Work out the finished part from the listing and answer in its coordinate system (mm). Give positions to 0.01 mm unless a question says otherwise; leave off trailing zeros. Loops run counter-clockwise (first coordinate to the right, second up) from the corner with the lowest first, then second, coordinate; pieces in that order, holes last. Notation, with made-up numbers: (28.5, 62.5) - (82.5, 62.5) arc R8 ccw to (82.5, 71.5) - close; hole circle Ø8 at (54.25, -30). An arc over 180 degrees is marked (long way). One line per question, with ' | ' between items.
Autodesk Inventor part; units mm, degrees
ref_plane "Work Plane1" through (9.2075, 0, 0) normal (1, 0, 0) x (0, 0, -1)
ref_plane "YZ Plane" through (0, 0, 0) normal (1, 0, 0) x (0, 1, 0)
ref_plane "XZ Plane" through (0, 0, 0) normal (0, 1, 0) x (-1, 0, 0)
sketch "Sketch1" plane through (0, 0, 0) normal (1, 0, 0) x (0, 1, 0)
  line L0 (147.32, 113.03) -> (-147.32, 113.03)
  line L1 (-147.32, 113.03) -> (-147.32, -113.03)
  line L2 (-147.32, -113.03) -> (147.32, -113.03)
  line L3 (147.32, -113.03) -> (147.32, 113.03)
  line L4 (147.32, 113.03) -> (-147.32, -113.03) construction
  line L5 (-147.32, 113.03) -> (147.32, -113.03) construction
  point P0 (0, 0)
  dimension "d0" = 294.64
  dimension "d1" = 226.06
extrude "Extrusion1" add sketch "Sketch1" along normal blind 2.8575
sketch "Sketch2" plane through (2.8575, 0, 0) normal (1, 0, 0) x (0, 0, -1)
  line L0 (113.03, 60.96) -> (100.33, 60.96)
  line L1 (100.33, 60.96) -> (100.33, -46.99)
  line L2 (100.33, -46.99) -> (113.03, -46.99)
  line L3 (113.03, -147.32) -> (113.03, 147.32)
  line L4 (113.03, 147.32) -> (-113.03, 147.32)
  line L5 (113.03, 60.96) -> (113.03, -46.99)
  point P0 (0, 0)
  dimension "d4" = 107.95
  dimension "d5" = 0
  dimension "d6" = 0
  dimension "d7" = 12.7
  dimension "d8" = 86.36
extrude "Extrusion2" cut sketch "Sketch2" against normal blind 2.8575
mirror "Mirror1" about plane through (0, 0, 0) normal (0, 0, 1) of "Extrusion2"
ref_plane "Work Plane1" through (9.2075, 0, 0) normal (1, 0, 0) x (0, 0, -1)
fillet "Fillet2" radius 0.762 12 edges at (0, 104.14, -113.03) (0, 6.985, -100.33) (0, 60.96, -106.68) (0, -97.155, -113.03) (0, -46.99, -106.68) (0, -147.32, 0) (0, -97.155, 113.03) (0, -46.99, 106.68) (0, 6.985, 100.33) (0, 60.96, 106.68) (0, 104.14, 113.03) (2.8575, 147.32, 0)
fillet "Fillet4" radius 0.254 18 edges at (2.8575, -147.32, 0) (2.8575, -97.155, -113.03) (2.8575, 6.985, -100.33) (2.8575, -46.99, -106.68) (2.6343, 147.0968, -113.03) (1.4287, 147.32, -113.03) (0.2232, 147.32, -112.8068) (0, 147.32, 0) (0.2232, 147.32, 112.8068) (1.4287, 147.32, 113.03) (2.6343, 147.0968, 113.03) (2.8575, 103.759, 113.03) (2.8575, 103.759, -113.03) (2.8575, 60.96, -106.68) (2.8575, 60.96, 106.68) (2.8575, 6.985, 100.33) (2.8575, -97.155, 113.03) (2.8575, -46.99, 106.68)
sketch "Sketch7" plane through (0, 0, 0) normal (-1, 0, 0) x (0, 0, 1)
  circle A0 centre (-13.97, -138.938) radius 2.54
  line L0 (0, 0) -> (0, -146.558) construction
  line L1 (112.268, -146.558) -> (-112.268, -146.558)
  circle A1 centre (13.97, -138.938) radius 2.54
  dimension "d22" = 5.08
  dimension "d23" = 13.97
  dimension "d24" = 7.62
extrude "Extrusion4" cut sketch "Sketch7" against normal up to next
properties part number "BackFlap"
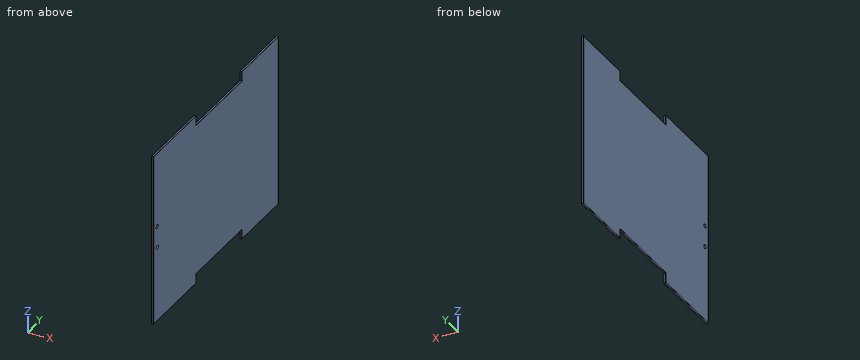
1. Find section A-A on y = 30. Write down the section's boundary in (x, z), then the cut area to 3 significant figures.
Evaluation:
outline: (0, -99.57) arc R0.76 ccw to (0.76, -100.33) - (2.6, -100.33) arc R0.25 ccw to (2.86, -100.08) - (2.86, 100.08) arc R0.25 ccw to (2.6, 100.33) - (0.76, 100.33) arc R0.76 ccw to (0, 99.57) - close | area: 573 mm2
2. Flat-ended cylindrical pins translate along their axes: pin 1 (0.6 mm diameter, centred on x = 1.5, y = -13, fed in from -Z); pin 2 (3 mm diameter, centred on y = -138.938, z = -13.97, fed in from +X). Find the tip coordinate at first contact, or state that the pin passes through.
Evaluation:
pin 1: z = -100.33 | pin 2: through
3. Consider L1, parallel to Y at x = 1.4, z = -13.97; L2, parallel to Z at x = 1.1, y = 36; L3, parallel to Y at x = 2.35, z = -16. Determine where each line is inside the solid, lowest interval first.
Evaluation:
L1: -147.32 to -141.48, -136.4 to 147.32 | L2: -100.33 to 100.33 | L3: -147.32 to -140.46, -137.41 to 147.28
